Work out the finished part from the listing and answer in its coordinate system (mm). A direction names the side the tool comes from. Round coordinates to 2 decimals unless told otherwise and drop trailing zeros. Loops run counter-clockwise (first coordinate to the right, second up) from the corner with the lowest first, then second, coordinate; pieces in that order, holes last.
```python
from build123d import *

# Parameters (mm, degrees)
ESQUISSE1_R             = 1.5
ESQUISSE1_R_2           = 4.5
BOSS_EXTRU_1_DEPTH      = 3
ESQUISSE2_W             = 22
ESQUISSE2_H             = 3
BOSS_EXTRU_2_DEPTH      = 22
ENL_V_MAT_EXTRU_1_REACH = 38.031
ESQUISSE3_R             = 1.5
CONG_1_R                = 4


with BuildPart() as part:
    # Esquisse1 → Boss.-Extru.1 (new body)
    with BuildSketch(Plane.XY):
        with BuildLine():
            Line((11, 0), (11, 15.5))
            Line((11, 15.5), (-11, 15.5))
            Line((-11, 15.5), (-11, 0))
            ThreePointArc((-11, 0), (0, -11), (11, 0))
        make_face()
        with Locations((8, 0)):
            Circle(ESQUISSE1_R, mode=Mode.SUBTRACT)
        with Locations((0, -8)):
            Circle(ESQUISSE1_R, mode=Mode.SUBTRACT)
        with Locations((0, 8)):
            Circle(ESQUISSE1_R, mode=Mode.SUBTRACT)
        with Locations((-8, 0)):
            Circle(ESQUISSE1_R, mode=Mode.SUBTRACT)
        Circle(ESQUISSE1_R_2, mode=Mode.SUBTRACT)
    extrude(amount=BOSS_EXTRU_1_DEPTH)

    # Esquisse2 → Boss.-Extru.2 (add)
    with BuildSketch(Plane.XY.offset(3)):
        with Locations((0, 14)):
            Rectangle(ESQUISSE2_W, ESQUISSE2_H)
    extrude(amount=BOSS_EXTRU_2_DEPTH)

    # Esquisse3 → Enlèv. mat.-Extru.1 (cut, up to next)
    with BuildSketch(Plane.XZ.offset(-12.5), mode=Mode.PRIVATE) as enl_v_mat_extru_1_sk1:
        with Locations((7, 21)):
            Circle(ESQUISSE3_R)
    enl_v_mat_extru_1_tool1 = extrude(enl_v_mat_extru_1_sk1.sketch, amount=-ENL_V_MAT_EXTRU_1_REACH, mode=Mode.PRIVATE) & part.part
    # Esquisse3 → Enlèv. mat.-Extru.1 (cut, up to next)
    with BuildSketch(Plane.XZ.offset(-12.5), mode=Mode.PRIVATE) as enl_v_mat_extru_1_sk2:
        with Locations((-7, 21)):
            Circle(ESQUISSE3_R)
    enl_v_mat_extru_1_tool2 = extrude(enl_v_mat_extru_1_sk2.sketch, amount=-ENL_V_MAT_EXTRU_1_REACH, mode=Mode.PRIVATE) & part.part
    # Esquisse3 → Enlèv. mat.-Extru.1 (cut, up to next)
    with BuildSketch(Plane.XZ.offset(-12.5), mode=Mode.PRIVATE) as enl_v_mat_extru_1_sk3:
        with Locations((7, 7)):
            Circle(ESQUISSE3_R)
    enl_v_mat_extru_1_tool3 = extrude(enl_v_mat_extru_1_sk3.sketch, amount=-ENL_V_MAT_EXTRU_1_REACH, mode=Mode.PRIVATE) & part.part
    # Esquisse3 → Enlèv. mat.-Extru.1 (cut, up to next)
    with BuildSketch(Plane.XZ.offset(-12.5), mode=Mode.PRIVATE) as enl_v_mat_extru_1_sk4:
        with Locations((-7, 7)):
            Circle(ESQUISSE3_R)
    enl_v_mat_extru_1_tool4 = extrude(enl_v_mat_extru_1_sk4.sketch, amount=-ENL_V_MAT_EXTRU_1_REACH, mode=Mode.PRIVATE) & part.part
    add(enl_v_mat_extru_1_tool1.solids().sort_by_distance((7, 12.5, 21))[0], mode=Mode.SUBTRACT)
    add(enl_v_mat_extru_1_tool2.solids().sort_by_distance((-7, 12.5, 21))[0], mode=Mode.SUBTRACT)
    add(enl_v_mat_extru_1_tool3.solids().sort_by_distance((7, 12.5, 7))[0], mode=Mode.SUBTRACT)
    add(enl_v_mat_extru_1_tool4.solids().sort_by_distance((-7, 12.5, 7))[0], mode=Mode.SUBTRACT)

    # Congé1
    cong_1_edges = [part.edges().sort_by_distance(p)[0] for p in [
        (11, 14, 25),
        (-11, 14, 25),
    ]]
    fillet(cong_1_edges, radius=CONG_1_R)


solid = part.part
```
1. Find section B-B (x = -8). Write down the section's boundary in (y, z).
Answer key:
outline: (-7.55, 0) - (-1.5, 0) - (-1.5, 3) - (-7.55, 3) - close; (1.5, 0) - (15.5, 0) - (15.5, 5.88) - (12.5, 5.88) - (12.5, 3) - (1.5, 3) - close; (12.5, 8.12) - (15.5, 8.12) - (15.5, 19.88) - (12.5, 19.88) - close; (12.5, 22.12) - (15.5, 22.12) - (15.5, 24.87) - (12.5, 24.87) - close
2. Which of the six approach directions +Z, -Z, +X, -X, +Y, -Y give full straight-line access (tool end or side, diameter ignored) to faces 4 (the face through (0, 6, 3)), 5 (the face through (5.89, 13.98, 22.01))?
Answer key:
face 4: +Z, +X, -X, -Y
face 5: +Y, -Y
3. Find section C-C (z = 7). Write down the section's boundary in (x, y), then the cut area to 3 significant figures.
Answer key:
outline: (-11, 12.5) - (-8.5, 12.5) - (-8.5, 15.5) - (-11, 15.5) - close; (-5.5, 12.5) - (5.5, 12.5) - (5.5, 15.5) - (-5.5, 15.5) - close; (8.5, 12.5) - (11, 12.5) - (11, 15.5) - (8.5, 15.5) - close
area: 48.0 mm2
4. Determine the mould class of faces 1 (the face through (11, 13, 6)), 2 (the face through (-0.325, -9.464, 1.479)), 3 (the face through (0, 15.5, 12)) for opening direction Y: +Y half, -Y half, draft (parallel to the pull), parting line (faces both ways), or undercut.
Answer key:
face 1: draft
face 2: undercut
face 3: +Y half
5. Consider probe 1 along Y at (x, z) = (0, 1.1); probe 2 along Z at (x, y) = (-7, 13.4); probe 3 along Y at (x, z) = (-7, 13.75). Determine where each line is inside the solid, lowest interval first.
Answer key:
probe 1: y = -11 to -9.5, -6.5 to -4.5, 4.5 to 6.5, 9.5 to 15.5
probe 2: z = 0 to 5.5, 8.5 to 19.5, 22.5 to 25
probe 3: y = 12.5 to 15.5
6. Find section D-D (x = -2.25). Write down the section's boundary in (y, z), then the cut area to 3 significant figures.
Answer key:
outline: (-10.77, 0) - (-3.9, 0) - (-3.9, 3) - (-10.77, 3) - close; (3.9, 0) - (15.5, 0) - (15.5, 25) - (12.5, 25) - (12.5, 3) - (3.9, 3) - close
area: 121 mm2
7. Given pin 1 (4 mm diameter, centred on x = 1, z = 10, fed in from -Y); pin 2 (1.8 mm diameter, centred on x = 8, y = 0, fed in from -Z); pin 3 (6 mm diameter, centred on x = -1, y = -5.5, fed in from +Z), each flat-ended and moving along its own axis, determine where each tip first touches the part or whether it passes through.
Answer key:
pin 1: stops at y = 12.5
pin 2: passes through
pin 3: stops at z = 3
8. Find section A-A (y = 8). Write down the section's boundary in (x, z), then the cut area to 3 significant figures.
Answer key:
outline: (-11, 0) - (-1.5, 0) - (-1.5, 3) - (-11, 3) - close; (1.5, 0) - (11, 0) - (11, 3) - (1.5, 3) - close
area: 57.0 mm2
